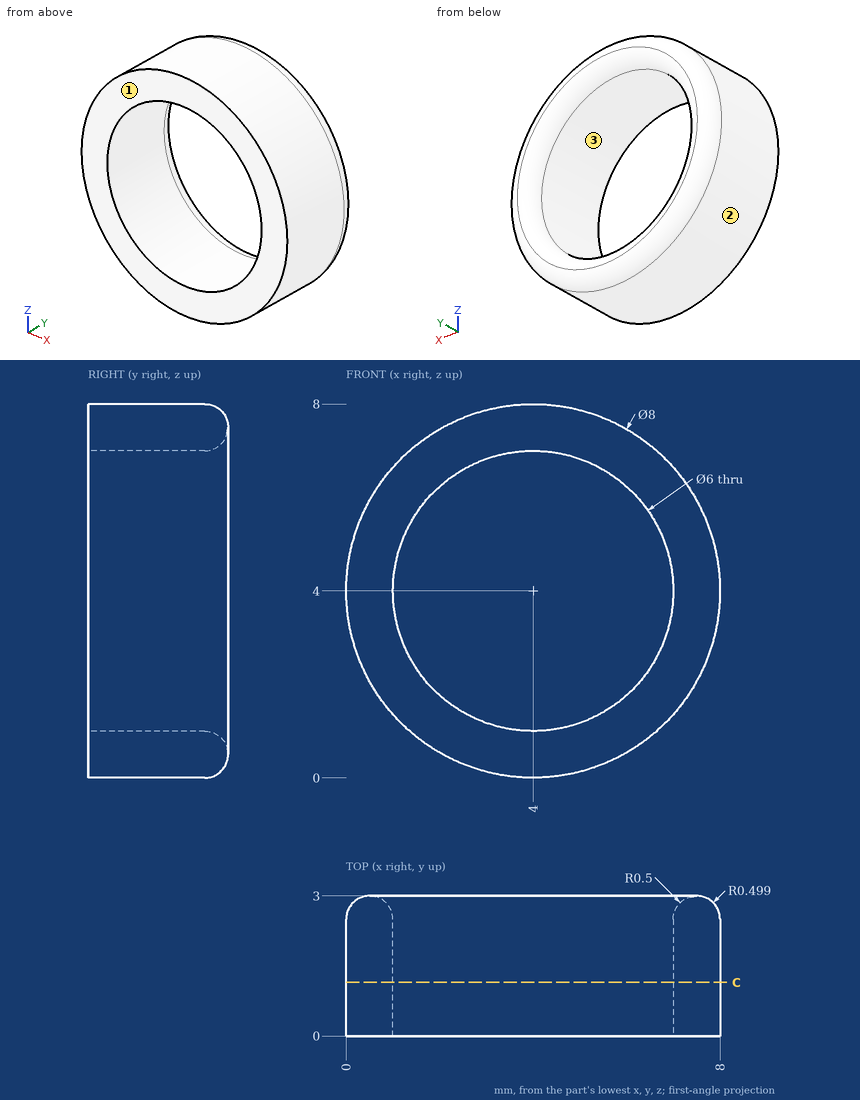
Answer from the drawing. Dimensions are ordinates in mm from the lowest x, y and z of the part. Give positions to 0.01 mm unless a question says otherwise; leave off trailing zeros. Order: outer loops, then holes, each group sorted by start corner. A loop starts at its lowest first (then second) coordinate and runs counter-clockwise, first axis right, second up. Notation, with made-up numbers: (51, -7) - (72, -7) arc R26 cw to (72, 29) - close; hole circle Ø4 at (0, -7). An arc over 180 degrees is marked (long way). One line per item, written item: value. Start each with the question number.
1) Find the intervals of material crossed by L1, parallel to Z at x = 4, y = 1.3; L2, parallel to X at y = 2.6, z = 1.75 (1 decimal); L3, parallel to Z at x = 6.5, y = 0.3 (1 decimal), in increasing order.
2) The mould has two halves that part along X. Classify the marked faces 1, 2 and 3: released by +X, released by -X, zero draft, split by the parting line, or undercut.
3) A cutting plane is placed at C-C on y = 1.15. Give the vertices of the cut face in (x, z).
4) Given pin 1 Ø1 at (y, z) = (2.5, 5.5) entering from -X; pin 2 Ø1 at (x, z) = (7, 7) entering from +Y, each flat-ended and moving along its own axis, determine where each tip first touches the part or whether it passes through.
Answer sheet:
1. L1: z = 0 to 1, 7 to 8
1. L2: x = 0.7 to 2, 6 to 7.3
1. L3: z = 0.9 to 2.3, 5.7 to 7.1
2. face 1: zero draft
2. face 2: split by the parting line
2. face 3: undercut
3. outline: circle Ø8 at (4, 4); hole circle Ø6 at (4, 4)
4. pin 1: stops at x = 0.13
4. pin 2: stops at y = 2.94
